Here's how the part is built. I have some questions about the finished solid (model axes, mm). Face numbers are marked on the shaded views. A direction names the side the tool comes from. Coordinates: 2 decimals unless noted, no trailing zeros. Write each loop counter-clockwise with the first axis right and the second up, starting at its lowest first coordinate (ties: lowest second). Pieces come first, ordered by that corner, then holes.
Item 1: I'm going to push flat-ended pins straight in: P1, Ø1.5, axis at x = 60, z = -41.5, coming from the +Y side; P2, Ø16.5, axis at x = 19, z = -21.5, coming from the +Y side. Where does each tip first touch, or does it pass through?
Item 2: Please list where these lines run through material, in increasing order: line 1 (X direction, y = 5, z = -3.2); line 2 (Z direction, x = 3, y = 6); line 3 (Z direction, x = 19.5, y = 5.5).
Item 3: For the marked faces 1 and 2, which set-ups out of +Z, -Z, +X, -X, +Y, -Y let a thin tool reach every point of the face, with its end or its side?
Item 4: I want a section at B-B (x = 48). Please give me the cut outline in (y, z).
Item 5: I want a section at D-D (x = 60.3). Please give me the cut outline in (y, z).
Item 6: If we mould it in two halves opening along Z, with no side actions, what happens to the marked faces 3, 4 and 5? For each: pulls with the +Z half, pulls with the -Z half, needs draft (parallel to the pull), parting line crosses it, or undercut.
Item 7: I want a section at A-A (y = 3). Please give me the cut outline in (x, z), and give its area (3 significant figures).
Item 8: I want a section at C-C (z = -3.2). Please give me the cut outline in (x, y).
from build123d import *

# Parameters (mm, degrees)
SKETCH1_W           = 63.5
SKETCH1_H           = 44.36533334
BOSS_EXTRUDE1_DEPTH = 7.8
SKETCH2_W           = 52.20000001
SKETCH2_H           = 33.06533334
CUT_EXTRUDE1_DEPTH  = 6.8
SKETCH3_R           = 1.5
SKETCH3_R_2         = 1.50000001
CUT_EXTRUDE2_DEPTH  = 7.5
FILLET1_R           = 2


with BuildPart() as part:
    # Sketch1 → Boss-Extrude1 (new body)
    with BuildSketch(Plane(origin=(0, 0, 0), x_dir=(1, 0, 0), z_dir=(0, 1, 0))):
        with Locations((31.75, 22.18266667)):
            Rectangle(SKETCH1_W, SKETCH1_H)
    extrude(amount=BOSS_EXTRUDE1_DEPTH)

    # Sketch2 → Cut-Extrude1 (cut)
    with BuildSketch(Plane(origin=(0, 7.8, 0), x_dir=(1, 0, 0), z_dir=(0, 1, 0))):
        with Locations((31.750000005, 22.18266667)):
            Rectangle(SKETCH2_W, SKETCH2_H)
    extrude(amount=-CUT_EXTRUDE1_DEPTH, mode=Mode.SUBTRACT)

    # Sketch3 → Cut-Extrude2 (cut)
    with BuildSketch(Plane(origin=(0, 7.8, 0), x_dir=(1, 0, 0), z_dir=(0, 1, 0))):
        with Locations(Location((3.2, 3.2, 0), (0, 0, 270))):
            Circle(SKETCH3_R)
        with Locations(Location((3.2, 41.16533334, 0), (0, 0, 270))):
            Circle(SKETCH3_R)
        with Locations(Location((60.3, 41.16533334, 0), (0, 0, 270))):
            Circle(SKETCH3_R_2)
        with Locations(Location((60.3, 3.2, 0), (0, 0, 270))):
            Circle(SKETCH3_R_2)
    extrude(amount=-CUT_EXTRUDE2_DEPTH, mode=Mode.SUBTRACT)

    # Fillet1
    fillet1_edges = [part.edges().sort_by_distance(p)[0] for p in [
        (0, 3.9, -44.36533334),
        (63.5, 3.9, -44.36533334),
        (63.5, 3.9, 0),
        (0, 3.9, 0),
    ]]
    fillet(fillet1_edges, radius=FILLET1_R)


solid = part.part
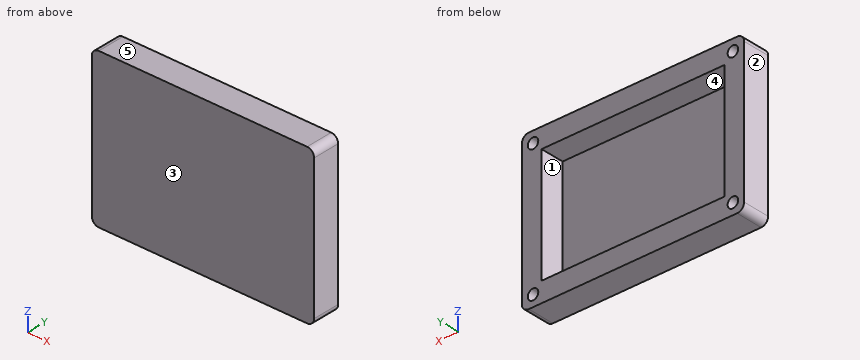
Answer:
1. P1: stops at y = 0.3
1. P2: stops at y = 1
2. line 1: x = 0 to 1.7, 4.7 to 58.8, 61.8 to 63.5
2. line 2: z = -44.37 to -42.65, -39.68 to -4.69, -1.71 to 0
2. line 3: z = -44.37 to -38.72, -5.65 to 0
3. face 1: +Y
3. face 2: +Z, -Z, -X, +Y, -Y
4. outline: (0, -44.37) - (7.8, -44.37) - (7.8, -38.72) - (1, -38.72) - (1, -5.65) - (7.8, -5.65) - (7.8, 0) - (0, 0) - close
5. outline: (0, -44.37) - (7.8, -44.37) - (7.8, -42.67) - (0.3, -42.67) - (0.3, -39.67) - (7.8, -39.67) - (7.8, -4.7) - (0.3, -4.7) - (0.3, -1.7) - (7.8, -1.7) - (7.8, 0) - (0, 0) - close
6. face 3: needs draft
6. face 4: undercut
6. face 5: pulls with the +Z half
7. outline: (0, -42.37) arc R2 ccw to (2, -44.37) - (61.5, -44.37) arc R2 ccw to (63.5, -42.37) - (63.5, -2) arc R2 ccw to (61.5, 0) - (2, 0) arc R2 ccw to (0, -2) - close; hole circle Ø3 at (3.2, -41.17); hole circle Ø3 at (3.2, -3.2); hole (5.65, -38.72) - (57.85, -38.72) - (57.85, -5.65) - (5.65, -5.65) - close; hole circle Ø3 at (60.3, -41.17); hole circle Ø3 at (60.3, -3.2)
7. area: 1,060 mm2
8. outline: (0, 0) - (63.5, 0) - (63.5, 7.8) - (61.8, 7.8) - (61.8, 0.3) - (58.8, 0.3) - (58.8, 7.8) - (4.7, 7.8) - (4.7, 0.3) - (1.7, 0.3) - (1.7, 7.8) - (0, 7.8) - close
